Source: CAD feature listing. Evaluate the final solid. Frame: model axes, mm. A direction names the side the tool comes from. Round coordinates to 2 decimals unless told otherwise and drop trailing zeros. Write each loop counter-clockwise with the first axis right and the second up, starting at its lowest first coordinate (ties: lowest second). Pieces come first, ordered by that corner, then holes.
from build123d import *


# Not quite as in the source:
# - a fillet or chamfer that OpenCascade refuses, or shapes differently, is made with other operations: its cross-section is extruded or revolved along the edge and cut away or added


with BuildPart() as f1:
    # F0 (on Top) → F1 (revolve)
    with BuildSketch(Plane.XY):
        Polygon((11.0400244594, -26.4020487666), (11.0400244594, 26.4020487666), (5.5200122297, 26.4020487666), (5.5200122297, 0), (5.5200122297, -26.4020487666), align=None)
        Polygon((0, 0), (5.5200122297, -26.4020487666), (5.5200122297, 0), align=None)
        Polygon((5.5200122297, 0), (5.5200122297, 26.4020487666), (0, 26.4020487666), align=None)
    revolve(axis=Axis((53.5406768322, 0, 0), (0, -1, 0)))

    # F2: fillet of radius 5 on 3 edges, made by hand

    # F2_s1 → F2_t2 (revolve, cut)
    with BuildSketch(Plane.XY):
        with BuildLine():
            ThreePointArc((6.1534879532, 26.4020487666), (2.2730077773, 24.5551224424), (1.2593119965, 20.3787982085))
            Line((1.2593119965, 20.3787982085), (0, 26.4020487666))
            Line((0, 26.4020487666), (6.1534879532, 26.4020487666))
        make_face()
    revolve(axis=Axis((53.5406768322, 26.4020487666, 0), (0, -1, 0)), mode=Mode.SUBTRACT)

    # F2_s3 → F2_t4 (revolve, cut)
    with BuildSketch(Plane.XY):
        with BuildLine():
            ThreePointArc((5.5200122297, 0), (2.0748843765, -2.0569822638), (1.2511057448, -5.9840003086))
            Line((1.2511057448, -5.9840003086), (0, 0))
            Line((0, 0), (5.5200122297, 0))
        make_face()
    revolve(axis=Axis((53.5406768322, 0, 0), (0, -1, 0)), mode=Mode.SUBTRACT)

    # F2_s5 → F2_t6 (revolve, cut)
    with BuildSketch(Plane.XY):
        with BuildLine():
            ThreePointArc((4.6885727551, -22.4252993247), (6.4296750361, -25.2825289425), (9.5827487118, -26.4020487666))
            Line((9.5827487118, -26.4020487666), (5.5200122297, -26.4020487666))
            Line((5.5200122297, -26.4020487666), (4.6885727551, -22.4252993247))
        make_face()
    revolve(axis=Axis((53.5406768322, -26.4020487666, 0), (0, -1, 0)), mode=Mode.SUBTRACT)


solid = f1.part
1) Pull-direction query (X, two-part tool) for faces 1 (the face through (36, 26.402, -39)), 2 (the face through (33.929, 0.37, 37.705)), 3 (the face through (30.921, -21.627, 43.488)); classes: released by +X, released by -X, zero draft, split by the parting line, or undercut.
Taken from the geometry:
face 1: zero draft
face 2: undercut
face 3: split by the parting line
2) Material intervals for line 1 (Z direction, x = 21, y = 6); line 2 (Z direction, x = 37, y = -18.5); line 3 (X direction, y = -5.5, z = -1.5), sorted ascending.
Taken from the geometry:
line 1: z = -37 to -27.34, 27.34 to 37
line 2: z = -46.84 to -39.15, 39.15 to 46.84
line 3: x = 1.2 to 11.07, 96.01 to 105.89
3) Section query B-B on y = -16. Return the cut outline in (x, z).
Taken from the geometry:
outline: circle Ø100.39 at (53.54, 0); hole circle Ø85 at (53.54, 0)
4) Section query A-A on z = 0. Return the cut outline in (x, y).
Taken from the geometry:
outline: (1.25, -5.98) - (4.69, -22.43) arc R5 ccw to (9.58, -26.4) - (11.04, -26.4) - (11.04, 26.4) - (6.15, 26.4) arc R5 ccw to (1.26, 20.38) - (5.52, 0) arc R5 ccw to start; (96.04, -26.4) - (97.5, -26.4) arc R5 ccw to (102.39, -22.43) - (105.83, -5.98) arc R5 ccw to (101.56, 0) - (105.82, 20.38) arc R5 ccw to (100.93, 26.4) - (96.04, 26.4) - close
5) Reachability of faces 4 (the face through (101.72, 0.99, -2.12)), 5 (the face through (77, -26.402, -36)) from +Z, -Z, +X, -X, +Y, -Y: full face, straight path, thin tool, end or side. Return the list, or none.
Taken from the geometry:
face 4: none
face 5: +Z, -Z, +X, -X, -Y
6) Contact query for flat-ended pins moving along their axis: P1, Ø1.5, axis at y = -8.5, z = -13, coming from the -X side; P2, Ø1, axis at y = -6.5, z = -21.5, coming from the -X side; P3, Ø3, axis at x = 76, y = 15.5, coming from the -Z side; P4, Ø5, axis at x = 80.5, z = 37, coming from the -Y side. Output: stop coordinate, or through.
Taken from the geometry:
P1: stops at x = 3.19
P2: stops at x = 5.74
P3: stops at z = -46.86
P4: stops at y = -26.4
